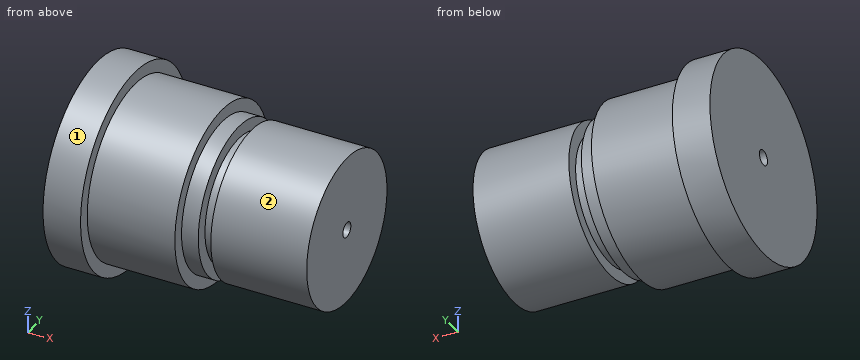
Autodesk Inventor part; units mm, degrees
ref_plane "YZ Plane" through (0, 0, 0) normal (1, 0, 0) x (0, 1, 0)
ref_plane "XZ Plane" through (0, 0, 0) normal (0, 1, 0) x (-1, 0, 0)
ref_plane "XY Plane" through (0, 0, 0) normal (0, 0, 1) x (1, 0, 0)
sketch "Эскиз1" plane through (0, 0, 0) normal (0, 0, 1) x (1, 0, 0)
  line L0 (0, 0) -> (100, 0)
  line L1 (100, 0) -> (100, 30)
  line L2 (100, 30) -> (50, 30)
  line L3 (50, 30) -> (50, 35)
  line L4 (50, 35) -> (15, 35)
  line L5 (15, 35) -> (15, 40)
  line L6 (15, 40) -> (0, 40)
  line L7 (0, 40) -> (0, 0)
  line L8 (56.6884, 30) -> (56.6884, 25)
  line L9 (56.6884, 25) -> (61.6884, 25)
  line L10 (61.6884, 25) -> (61.6884, 30)
  dimension "d0" = 100
  dimension "d1" = 30
  dimension "d2" = 50
  dimension "d3" = 5
  dimension "d4" = 35
  dimension "d5" = 5
  dimension "d7" = 5
  dimension "d8" = 5
  dimension "d9" = 11.6884
revolve "Вращение1" add sketch "Эскиз1" angle 360 about axis through (0, 0, 0) along (1, 0, 0)
revolve "Вращение2" cut sketch "Эскиз1" angle 360 about axis through (0, 0, 0) along (-1, 0, 0) contours L10 L9 L8 L2
sketch "Эскиз2" plane through (0, 0, 0) normal (1, 0, 0) x (0, 1, 0)
  circle A0 centre (0, 0) radius 3
  dimension "d11" = 6
extrude "Выдавливание1" cut sketch "Эскиз2" along normal up to surface (100 mm away)
properties part number "1"
The model under review builds one solid part; all positions refer to its coordinate system, in mm. Face numbers are marked on the shaded views. A direction names the side the tool comes from. Round coordinates to 2 decimals unless told otherwise and drop trailing zeros. Order: outer loops, then holes, each group sorted by start corner. A loop starts at its lowest first (then second) coordinate and runs counter-clockwise, first axis right, second up. Notation, with made-up numbers: M -14,-30 L -10,-30 A18 cw -10,-5 Z; hole C -17.5,-35.75 d11. An arc over 180 degrees is marked long. Use a Markdown table: item, result.
1) Consider section A-A (y = 0). Write out the cut boundary in (x, z).
Report:
| item | result |
|---|---|
| outline | M 0,-40 L 15,-40 L 15,-35 L 50,-35 L 50,-30 L 56.69,-30 L 56.69,-25 L 61.69,-25 L 61.69,-30 L 100,-30 L 100,-3 L 0,-3 Z; M 0,3 L 100,3 L 100,30 L 61.69,30 L 61.69,25 L 56.69,25 L 56.69,30 L 50,30 L 50,35 L 15,35 L 15,40 L 0,40 Z |
2) Insertion check: pin 1 (1 mm diameter, centred on x = 76.5, z = -28, fed in from +Y); pin 2 (3 mm diameter, centred on x = 54.5, z = 20.5, fed in from +Y); pin 3 (12 mm diameter, centred on x = 79, z = 27, fed in from +Y). Each pin has a flat end and moves straight along its axis. Give the tip position at first contact, or say it passes through.
Report:
| item | result |
|---|---|
| pin 1 | y = 11.99 |
| pin 2 | y = 23.22 |
| pin 3 | y = 21.42 |
3) Consider section C-C (x = 37). Write out the cut boundary in (y, z).
Report:
| item | result |
|---|---|
| outline | C 0,0 d70; hole C 0,0 d6 |
4) Wall thickness on line 1 along Z through (x, y) = (60, 0); line 2 along Z through (x, y) = (72, 0); line 3 along X through (y, z) = (-3, 33.5): over which ranges is each line inside the solid? List them lowest first. Write a range as [from, to].
Report:
| item | result |
|---|---|
| line 1 | [-25, -3], [3, 25] |
| line 2 | [-30, -3], [3, 30] |
| line 3 | [0, 50] |
5) Consider section D-D (z = 23.5). Write out the cut boundary in (x, y), then the cut area to 3 significant figures.
Report:
| item | result |
|---|---|
| outline | M 0,-32.37 L 15,-32.37 L 15,-25.94 L 50,-25.94 L 50,-18.65 L 56.69,-18.65 L 56.69,-8.53 L 61.69,-8.53 L 61.69,-18.65 L 100,-18.65 L 100,18.65 L 61.69,18.65 L 61.69,8.53 L 56.69,8.53 L 56.69,18.65 L 50,18.65 L 50,25.94 L 15,25.94 L 15,32.37 L 0,32.37 Z |
| area | 4,550 mm^2 |
6) Tool access review of the marked faces 1 and 2: name each direction out of +Z, -Z, +X, -X, +Y, -Y from which nothing blocks a thin tool from reaching the whole face with its end or side.
Report:
| item | result |
|---|---|
| face 1 | +X, -X |
| face 2 | +X |
